Source: three-view drawing plus pictorial views. Frame: mm from the lowest corner of the part. Give positions to 0.01 mm unless a question says otherwise; leave off trailing zeros. Loops run counter-clockwise (first coordinate to the right, second up) from the corner with the lowest first, then second, coordinate; pieces in that order, holes last.
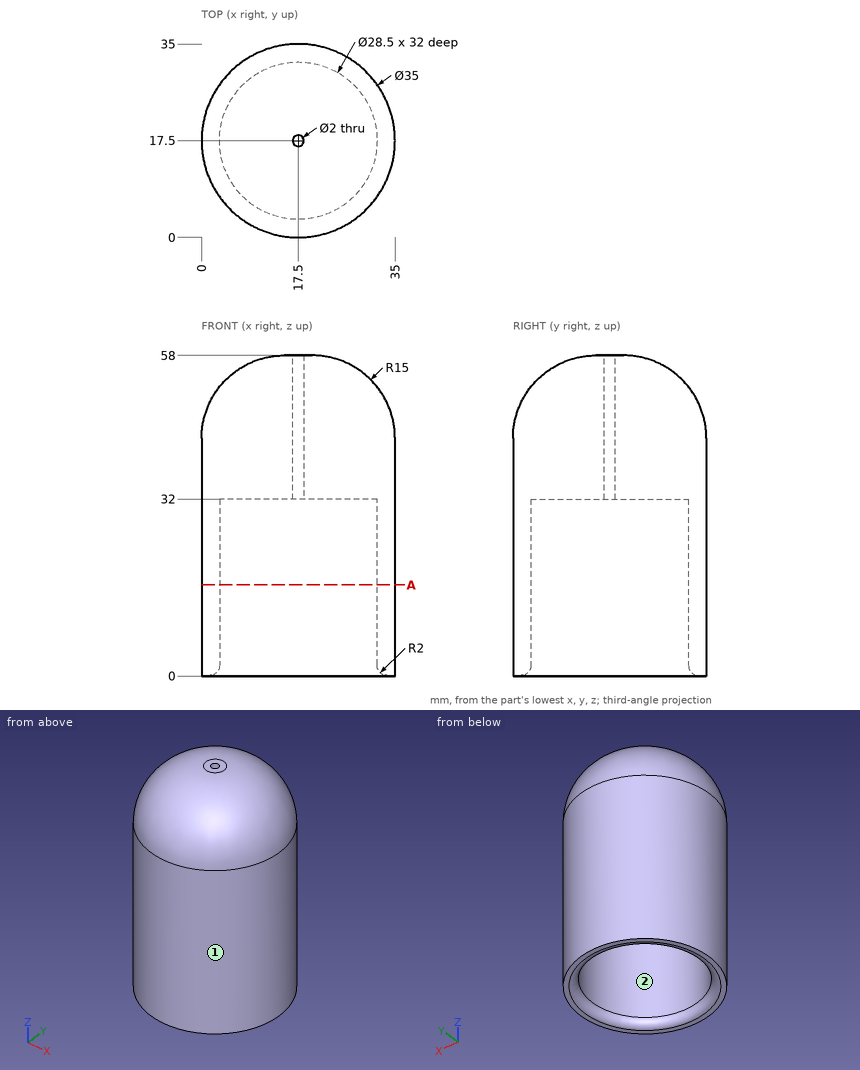
(1) Cut plane A-A (z = 16.5). Return the cut outline in (x, y), and give its area (3 significant figures).
Values follow:
outline: circle Ø35 at (17.5, 17.5); hole circle Ø28.5 at (17.5, 17.5)
area: 324 mm2
(2) Ray query, probe 1 along Y at (x, z) = (17.5, 38.75); probe 2 along X at (y, z) = (17, 25); probe 3 along Y at (x, z) = (17.5, 20). Return the intervals inside material, ascending.
Values follow:
probe 1: y = 0 to 16.5, 18.5 to 35
probe 2: x = 0.01 to 3.26, 31.74 to 34.99
probe 3: y = 0 to 3.25, 31.75 to 35
(3) Mould query, pull axis Y, two halves, no side actions, for the marked faces 1 and 2. Classes: +Y half, -Y half, draft (parallel to the pull), parting line (faces both ways), or undercut.
Values follow:
face 1: parting line
face 2: undercut
(4) Pin query (flat end, axial travel): pin 1 Ø5 at (y, z) = (11.5, 17.5) entering from -X; pin 2 Ø10 at (y, z) = (8, 33) entering from -X; pin 3 Ø5 at (x, y) = (15.5, 12.5) entering from +Z; pin 4 Ø12 at (y, z) = (15, 42.5) entering from +X. Return the tip coordinate at first contact, or that it passes through.
Values follow:
pin 1: stops at x = 0.35
pin 2: stops at x = 0.59
pin 3: stops at z = 58
pin 4: stops at x = 35
